```python
from build123d import *

# Parameters (mm, degrees)
SKETCH_W        = 30
SKETCH_H        = 78.5
SKETCH_W_2      = 20
SKETCH_H_2      = 40.5
PAD_DEPTH       = 5
SKETCH001_W     = 30
SKETCH001_H     = 8
PAD004_DEPTH    = 47
SKETCH002_W     = 5
SKETCH002_H     = 8
PAD005_DEPTH    = 31
PAD006_DEPTH    = 8
SKETCH006_R     = 1.5
POCKET001_DEPTH = 6.501
SKETCH007_R     = 5.75
POCKET002_DEPTH = 30.001


with BuildPart() as part:
    # Sketch → Pad (new body)
    with BuildSketch(Plane.YZ):
        with Locations((10, 9.25)):
            Rectangle(SKETCH_W, SKETCH_H)
        with Locations((10, 20.25)):
            Rectangle(SKETCH_W_2, SKETCH_H_2, mode=Mode.SUBTRACT)
    extrude(amount=-PAD_DEPTH)

    # Sketch001 → Pad004 (join)
    with BuildSketch(Plane.YZ):
        with Locations((10, -26)):
            Rectangle(SKETCH001_W, SKETCH001_H)
    extrude(amount=PAD004_DEPTH)

    # Sketch002 → Pad005 (join)
    with BuildSketch(Plane.YZ):
        with Locations((-2.5, 44.5)):
            Rectangle(SKETCH002_W, SKETCH002_H)
        with Locations((22.5, 44.5)):
            Rectangle(SKETCH002_W, SKETCH002_H)
    extrude(amount=PAD005_DEPTH)

    # Sketch003 → Pad006 (join)
    with BuildSketch(Plane.XY.offset(40.5)):
        with BuildLine():
            ThreePointArc((34, 15), (29, 10), (34, 5))
            Line((34, 5), (34, -5))
            Line((34, -5), (31, -5))
            Line((31, -5), (31, 2.583802))
            ThreePointArc((31, 17.416198), (26, 10), (31, 2.583802))
            Line((31, 25), (31, 17.416198))
            Line((34, 25), (31, 25))
            Line((34, 15), (34, 25))
        make_face()
    extrude(amount=PAD006_DEPTH)

    # Sketch006 → Pocket001 (cut, through all)
    with BuildSketch(Plane.YZ.offset(40.5)):
        with Locations((-2.5, 44.5)):
            Circle(SKETCH006_R)
        with Locations((22.5, 44.5)):
            Circle(SKETCH006_R)
    extrude(amount=POCKET001_DEPTH, mode=Mode.SUBTRACT)

    # Sketch007 → Pocket002 (cut, through all)
    with BuildSketch(Plane.XY):
        with Locations((34, 10)):
            Circle(SKETCH007_R)
    extrude(amount=-POCKET002_DEPTH, mode=Mode.SUBTRACT)


solid = part.part
```
Design review of the part built by this model. Coordinates are the model's own, in mm. A direction names the side the tool comes from. Give positions to 0.01 mm unless a question says otherwise; leave off trailing zeros. Write each loop counter-clockwise with the first axis right and the second up, starting at its lowest first coordinate (ties: lowest second). Pieces come first, ordered by that corner, then holes.
(1) Tool access review of faces 5 (the face through (31, 19, 44)), 6 (the face through (34, 0, 44)), 7 (the face through (21, 20.2, 40.5)), 8 (the face through (-2, 0, 20)): name each direction out of +Z, -Z, +X, -X, +Y, -Y from which nothing blocks a thin tool from reaching the whole face with its end or side.
Checked values:
face 5: +Z
face 6: +Z, +X, +Y, -Y
face 7: +X, +Y, -Y
face 8: +X, -X
(2) Clearance check with flat-ended pins moving along their axes: pin 1 Ø15 at (y, z) = (14.5, 16.5) entering from +X; pin 2 Ø2.5 at (y, z) = (-0.5, 45) entering from +X. State where each tip first meets the part, or that it passes through.
Checked values:
pin 1: stops at x = 0
pin 2: stops at x = 34
(3) Wall thickness on line 1 along Y through (x, z) = (34, -25.5); line 2 along Z through (x, y) = (31, -0.75); line 3 along Z through (x, y) = (12.5, 19): over which ranges is each line inside the solid? List them lowest first.
Checked values:
line 1: y = -5 to 4.25, 15.75 to 25
line 2: z = -30 to -22, 40.5 to 48.5
line 3: z = -30 to -22
(4) Add section C-C (y = 21). Give the boundary of the cut face in (x, z).
Checked values:
outline: (-5, -30) - (47, -30) - (47, -22) - (0, -22) - (0, 40.5) - (34, 40.5) - (34, 48.5) - (-5, 48.5) - close
(5) Mouldability with a two-part tool opening along Z and no side actions: class faces 1 (the face through (34, 20, 44)), 2 (the face through (14.8, 20.2, 48.5)), 3 (the face through (21, 10, -30)), 4 (the face through (-2, 20, 20)) as +Z half, -Z half, draft (parallel to the pull), parting line (faces both ways), or undercut.
Checked values:
face 1: draft
face 2: +Z half
face 3: -Z half
face 4: undercut
(6) Add section B-B (y = 10). Give the boundary of the cut face in (x, z).
Checked values:
outline: (-5, -30) - (28.25, -30) - (28.25, -22) - (0, -22) - (0, 0) - (-5, 0) - close; (-5, 40.5) - (0, 40.5) - (0, 48.5) - (-5, 48.5) - close; (26, 40.5) - (29, 40.5) - (29, 48.5) - (26, 48.5) - close; (39.75, -30) - (47, -30) - (47, -22) - (39.75, -22) - close
(7) Add section D-D (z = -5.5). Give the boundary of the cut face in (x, y).
Checked values:
outline: (-5, -5) - (0, -5) - (0, 25) - (-5, 25) - close
(8) Add section A-A (z = 14). Give the boundary of the cut face in (x, y), and give its area (3 significant figures).
Checked values:
outline: (-5, -5) - (0, -5) - (0, 0) - (-5, 0) - close; (-5, 20) - (0, 20) - (0, 25) - (-5, 25) - close
area: 50.0 mm2
